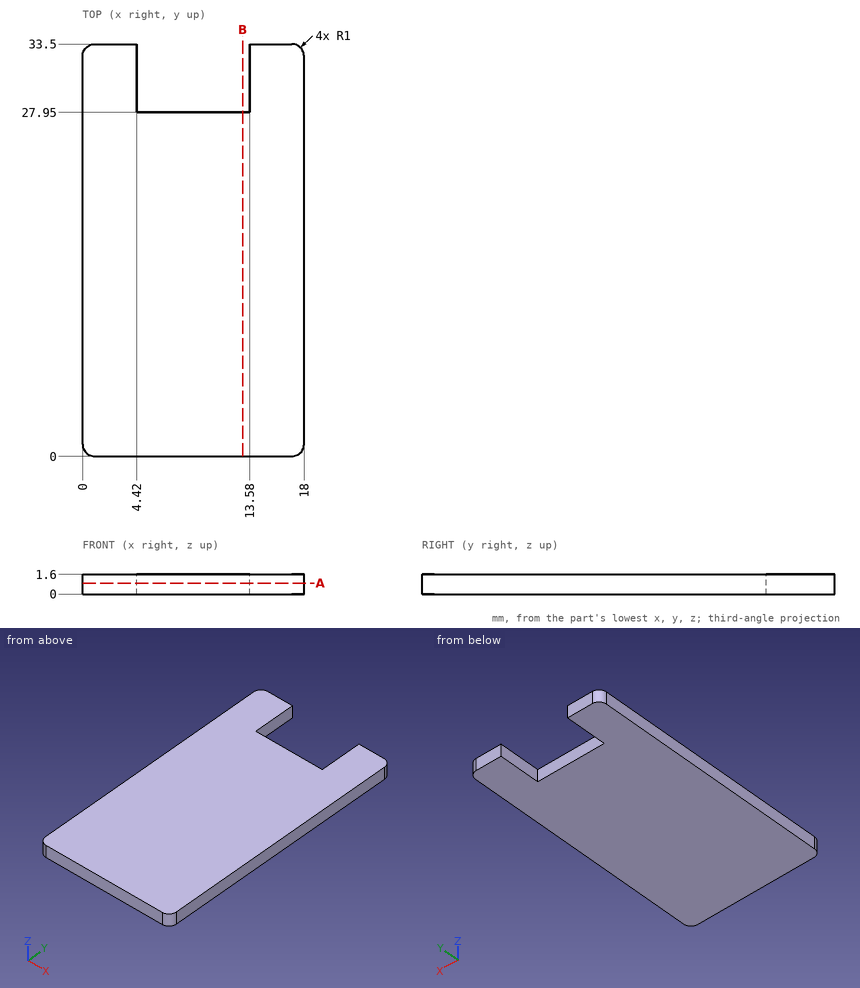
Design review of the part shown in the three views and the two pictorial views. Dimensions are in mm from the part's minimum x, y and z. Round coordinates to 2 decimals unless told otherwise and drop trailing zeros. Write each loop counter-clockwise with the first axis right and the second up, starting at its lowest first coordinate (ties: lowest second). Pieces come first, ordered by that corner, then holes. Notation, with made-up numbers: M -31,67 L 8,67 A31 cw 8,95 Z; hole C 22.5,33.25 d10. An arc over 180 degrees is marked long. Use a Markdown table: item, result. Add a question column.
Q1. We need section A-A, the plane z = 0.9. State the section outline as (x, y) points.
Q2. To check wall thickness, follow line 1 (X direction, y = 28, z = 0.2); line 2 (Y direction, x = 13, z = 0.6). State the ranges of each line that lie inside material, in increasing order.
Q3. We need section B-B, the plane x = 13. State the section outline as (y, z) points, plus the area to 3 significant figures.
Q4. Insertion check: pin 1 (0.5 mm diameter, centred on x = 9.5, z = 0.5, fed in from +Y). The pin has a flat end and moves straight along its axis. Give the tip position at first contact, or say it passes through.
Findings below:
| question | item | result |
|---|---|---|
| 1 | outline | M 0,1 A1 ccw 1,0 L 17,0 A1 ccw 18,1 L 18,32.5 A1 ccw 17,33.5 L 13.58,33.5 L 13.58,27.95 L 4.42,27.95 L 4.42,33.5 L 1,33.5 A1 ccw 0,32.5 Z |
| 2 | line 1 | x = 0 to 4.42, 13.58 to 18 |
| 2 | line 2 | y = 0 to 27.95 |
| 3 | outline | M 0,0 L 27.95,0 L 27.95,1.6 L 0,1.6 Z |
| 3 | area | 44.7 mm² |
| 4 | pin 1 | stops at y = 27.95 |
